Design review of the part built by this model. Coordinates are the model's own, in mm. A direction names the side the tool comes from. Round coordinates to 2 decimals unless told otherwise and drop trailing zeros. Loops run counter-clockwise (first coordinate to the right, second up) from the corner with the lowest first, then second, coordinate; pieces in that order, holes last. Notation, with made-up numbers: (-22.75, -12) - (31.25, -12) arc R19 cw to (31.25, -4) - close; hole circle Ø11 at (-34, -24.5). An arc over 180 degrees is marked (long way). Use one line per item in the form item = value. Start each with the question number.
(1) We need section B-B, the plane x = 14. Write out the cut boundary in (y, z), then the cut area to 3 significant figures.
(2) Wall thickness on probe 1 along X at (y, z) = (-2, 0); probe 2 along X at (y, z) = (1.5, 2.25); probe 3 along Y at (x, z) = (15, -5.25): over which ranges is each line inside the solid? List them lowest first. Write a range as [from, to].
(3) Machinability: for faces 1 (the flat face through (0, -6.678, 0)), 2 (the flat face through (0, -4.9, -7)), 3 (the flat face through (0, -6, 3)), which of the approach directions +Z, -Z, +X, -X, +Y, -Y give a long, thin tool a straight path to every point of the face, cutting with its end or side? Answer none if there is none.
(4) We need section C-C, the plane x = -1. Write out the cut boundary in (y, z), then the cut area to 3 significant figures.
(5) For pin 1 (2 mm diameter, centred on x = -4.5, z = -6, fed in from -Y); pin 2 (0.9 mm diameter, centred on x = 3, y = -6, fed in from +Z); pin 3 (0.5 mm diameter, centred on x = 5, y = -6, fed in from -Z), all flat-tipped, find the tip position at first contact; note any pin that passes through.
(6) The part is to be moulded in two halves that separate along X. For faces 4 (the flat face through (20, -1, 0)), 5 (the cylindrical face through (-11.834, -0.808, -0.338)), 6 (the cylindrical face through (12.105, -0.808, 1.2)), 7 (the flat face through (0, -6, -3)), say which applies: released by +X, released by -X, zero draft, split by the parting line, or undercut.
(7) We need section D-D, the plane y = 1. Write out the cut boundary in (x, z), then the cut area to 3 significant figures.
(8) We need section A-A, the plane z = 0. Write out the cut boundary in (x, y).
from build123d import *

# Parameters (mm, degrees)
BOSS_EXTRUDE1_DEPTH = 20
SKETCH2_R           = 2.6
CUT_EXTRUDE1_DEPTH  = 11.578
FILLET1_R           = 2.54


with BuildPart() as part:
    # Sketch1 → Boss-Extrude1 (new, symmetric)
    with BuildSketch(Plane(origin=(0, 0, 0), x_dir=(0, 0, -1), z_dir=(1, 0, 0))):
        Polygon((-10, 4.9), (10, 4.9), (10, -4.9), (3, -4.9), (3, -6.678), (-3, -6.678), (-3, -4.9), (-10, -4.9), align=None)
    extrude(amount=BOSS_EXTRUDE1_DEPTH, both=True)

    # Sketch2 → Cut-Extrude1 (cut)
    with BuildSketch(Plane(origin=(0, 4.9, 0), x_dir=(1, 0, 0), z_dir=(0, 1, 0))):
        with Locations(Location((-14.412, 0, 0), (0, 0, 270))):
            Circle(SKETCH2_R)
        with Locations(Location((14.412, 0, 0), (0, 0, 270))):
            Circle(SKETCH2_R)
    extrude(amount=-CUT_EXTRUDE1_DEPTH, mode=Mode.SUBTRACT)

    # Fillet1
    fillet1_edges = [part.edges().sort_by_distance(p)[0] for p in [
        (-20, 0, -10),
        (20, 0, 10),
        (20, 0, -10),
        (-20, 0, 10),
    ]]
    fillet(fillet1_edges, radius=FILLET1_R)


solid = part.part
Data:
q1.outline = (-6.68, -3) - (-4.9, -3) - (-4.9, -10) - (4.9, -10) - (4.9, -2.57) - (-6.68, -2.57) - close; (-6.68, 2.57) - (4.9, 2.57) - (4.9, 10) - (-4.9, 10) - (-4.9, 3) - (-6.68, 3) - close
q1.area = 147 mm^2
q2.probe_1 = [-20, -17.01], [-11.81, 11.81], [17.01, 20]
q2.probe_2 = [-20, -15.71], [-13.11, 13.11], [15.71, 20]
q2.probe_3 = [-4.9, 4.9]
q3.face_1 = +Z, -Z, +X, -X, -Y
q3.face_2 = -Z, +X, -X, -Y
q3.face_3 = +Z, +X, -X, -Y
q4.outline = (-6.68, -3) - (-4.9, -3) - (-4.9, -10) - (4.9, -10) - (4.9, 10) - (-4.9, 10) - (-4.9, 3) - (-6.68, 3) - close
q4.area = 207 mm^2
q5.pin_1 = -4.9
q5.pin_2 = 3
q5.pin_3 = -3
q6.face_4 = released by +X
q6.face_5 = undercut
q6.face_6 = undercut
q6.face_7 = zero draft
q7.outline = (-20, -7.46) arc R2.54 ccw to (-17.46, -10) - (17.46, -10) arc R2.54 ccw to (20, -7.46) - (20, 7.46) arc R2.54 ccw to (17.46, 10) - (-17.46, 10) arc R2.54 ccw to (-20, 7.46) - close; hole circle Ø5.2 at (-14.41, 0); hole circle Ø5.2 at (14.41, 0)
q7.area = 752 mm^2
q8.outline = (-20, -6.68) - (-17.01, -6.68) - (-17.01, 4.9) - (-20, 4.9) - close; (-11.81, -6.68) - (11.81, -6.68) - (11.81, 4.9) - (-11.81, 4.9) - close; (17.01, -6.68) - (20, -6.68) - (20, 4.9) - (17.01, 4.9) - close
